Check sheet for the modelled part. Datum: model origin and axes. Units: mm. Round coordinates to 2 decimals unless told otherwise and drop trailing zeros. Loops run counter-clockwise (first coordinate to the right, second up) from the corner with the lowest first, then second, coordinate; pieces in that order, holes last. Notation, with made-up numbers: (74, -40) -> (116, -40) arc R11 ccw to (116, -36) -> close; hole circle Ø4 at (6, 60.25). An arc over 180 degrees is marked (long way). One line per item, written item: value. Start each with the question number.
1. Cross-section at A-A on y = -41.05. Record the cut outline in (x, z), then the cut area to 3 significant figures.
2. Go/stop test with a flat-tipped pin: pin 1 (2.5 mm diameter, centred on x = 5, y = -41.05, fed in from -Z). Record where the tip stops, or that it passes through.
3. Cross-section at C-C on x = 50. Record the cut outline in (y, z), then the cut area to 3 significant figures.
4. Material ranges on L1, parallel to Y at x = 32.55, z = 0.85; L2, parallel to X at y = -76.1, z = 1.15; L3, parallel to Y at x = 21, z = 0.6, recorded low to high.
5. Cross-section at B-B on x = 60.1. Record the cut outline in (y, z).
6. Cross-section at D-D on x = 29. Record the cut outline in (y, z).
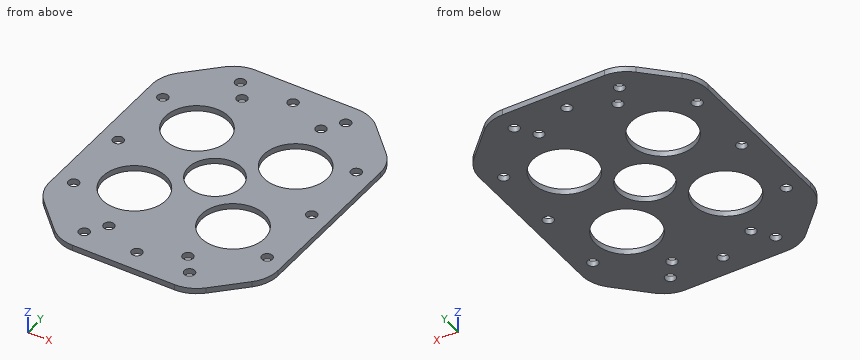
from build123d import *

# Parameters (mm, degrees)
IZIM1_R                     = 9
IZIM1_R_2                   = 7.55
IZIM1_R_3                   = 1.5
Y_KSEKLIK_EKSTR_ZYON1_DEPTH = 1.6


with BuildPart() as part:
    # Çizim1 → Yükseklik-Ekstrüzyon1 (new body)
    with BuildSketch(Plane.XY):
        with BuildLine():
            Line((2.928932188, -10.971067812), (10.971067812, -2.928932188))
            ThreePointArc((10.971067812, -2.928932188), (14.2153013, -0.761204675), (18.042135624, 0))
            Line((18.042135624, 0), (47.057864376, 0))
            ThreePointArc((47.057864376, 0), (50.8846987, -0.761204675), (54.128932188, -2.928932188))
            Line((54.128932188, -2.928932188), (62.171067812, -10.971067812))
            ThreePointArc((62.171067812, -10.971067812), (64.338795325, -14.2153013), (65.1, -18.042135624))
            Line((65.1, -18.042135624), (65.1, -64.057864376))
            ThreePointArc((65.1, -64.057864376), (64.338795325, -67.8846987), (62.171067812, -71.128932188))
            Line((62.171067812, -71.128932188), (54.128932188, -79.171067812))
            ThreePointArc((54.128932188, -79.171067812), (50.8846987, -81.338795325), (47.057864376, -82.1))
            Line((47.057864376, -82.1), (18.042135624, -82.1))
            ThreePointArc((18.042135624, -82.1), (14.2153013, -81.338795325), (10.971067812, -79.171067812))
            Line((10.971067812, -79.171067812), (2.928932188, -71.128932188))
            ThreePointArc((2.928932188, -71.128932188), (0.761204675, -67.8846987), (0, -64.057864376))
            Line((0, -64.057864376), (0, -18.042135624))
            ThreePointArc((0, -18.042135624), (0.761204675, -14.2153013), (2.928932188, -10.971067812))
        make_face()
        with Locations((18.5, -27)):
            Circle(IZIM1_R, mode=Mode.SUBTRACT)
        with Locations((46.6, -27)):
            Circle(IZIM1_R, mode=Mode.SUBTRACT)
        with Locations((18.5, -55.1)):
            Circle(IZIM1_R, mode=Mode.SUBTRACT)
        with Locations((46.6, -55.1)):
            Circle(IZIM1_R, mode=Mode.SUBTRACT)
        with Locations((32.55, -41.05)):
            Circle(IZIM1_R_2, mode=Mode.SUBTRACT)
        with Locations((32.55, -6)):
            Circle(IZIM1_R_3, mode=Mode.SUBTRACT)
        with Locations((47.55, -6)):
            Circle(IZIM1_R_3, mode=Mode.SUBTRACT)
        with Locations((43.8, -11.2)):
            Circle(IZIM1_R_3, mode=Mode.SUBTRACT)
        with Locations((17.55, -6)):
            Circle(IZIM1_R_3, mode=Mode.SUBTRACT)
        with Locations((21.3, -11.2)):
            Circle(IZIM1_R_3, mode=Mode.SUBTRACT)
        with Locations((5, -21.05)):
            Circle(IZIM1_R_3, mode=Mode.SUBTRACT)
        with Locations((60.1, -21.05)):
            Circle(IZIM1_R_3, mode=Mode.SUBTRACT)
        with Locations((5, -41.05)):
            Circle(IZIM1_R_3, mode=Mode.SUBTRACT)
        with Locations((60.1, -41.05)):
            Circle(IZIM1_R_3, mode=Mode.SUBTRACT)
        with Locations(Location((60.1, -61.05, 0), (0, 0, 180))):
            Circle(IZIM1_R_3, mode=Mode.SUBTRACT)
        with Locations(Location((32.55, -76.1, 0), (0, 0, 180))):
            Circle(IZIM1_R_3, mode=Mode.SUBTRACT)
        with Locations(Location((47.55, -76.1, 0), (0, 0, 180))):
            Circle(IZIM1_R_3, mode=Mode.SUBTRACT)
        with Locations(Location((43.8, -70.9, 0), (0, 0, 180))):
            Circle(IZIM1_R_3, mode=Mode.SUBTRACT)
        with Locations(Location((21.3, -70.9, 0), (0, 0, 180))):
            Circle(IZIM1_R_3, mode=Mode.SUBTRACT)
        with Locations(Location((17.55, -76.1, 0), (0, 0, 180))):
            Circle(IZIM1_R_3, mode=Mode.SUBTRACT)
        with Locations(Location((5, -61.05, 0), (0, 0, 180))):
            Circle(IZIM1_R_3, mode=Mode.SUBTRACT)
    extrude(amount=Y_KSEKLIK_EKSTR_ZYON1_DEPTH)


solid = part.part
Taken from the geometry:
1. outline: (0, 0) -> (3.5, 0) -> (3.5, 1.6) -> (0, 1.6) -> close; (6.5, 0) -> (25, 0) -> (25, 1.6) -> (6.5, 1.6) -> close; (40.1, 0) -> (58.6, 0) -> (58.6, 1.6) -> (40.1, 1.6) -> close; (61.6, 0) -> (65.1, 0) -> (65.1, 1.6) -> (61.6, 1.6) -> close
1. area: 70.4 mm2
2. pin 1: passes through
3. outline: (-81.66, 0) -> (-63.43, 0) -> (-63.43, 1.6) -> (-81.66, 1.6) -> close; (-46.77, 0) -> (-35.33, 0) -> (-35.33, 1.6) -> (-46.77, 1.6) -> close; (-18.67, 0) -> (-0.44, 0) -> (-0.44, 1.6) -> (-18.67, 1.6) -> close
3. area: 76.6 mm2
4. L1: y = -82.1 to -77.6, -74.6 to -48.6, -33.5 to -7.5, -4.5 to 0
4. L2: x = 7.9 to 16.05, 19.05 to 31.05, 34.05 to 46.05, 49.05 to 57.2
4. L3: y = -82.1 to -72.37, -69.43 to -63.75, -46.45 to -35.65, -18.35 to -12.67, -9.73 to 0
5. outline: (-73.2, 0) -> (-62.55, 0) -> (-62.55, 1.6) -> (-73.2, 1.6) -> close; (-59.55, 0) -> (-42.55, 0) -> (-42.55, 1.6) -> (-59.55, 1.6) -> close; (-39.55, 0) -> (-22.55, 0) -> (-22.55, 1.6) -> (-39.55, 1.6) -> close; (-19.55, 0) -> (-8.9, 0) -> (-8.9, 1.6) -> (-19.55, 1.6) -> close
6. outline: (-82.1, 0) -> (-47.71, 0) -> (-47.71, 1.6) -> (-82.1, 1.6) -> close; (-34.39, 0) -> (0, 0) -> (0, 1.6) -> (-34.39, 1.6) -> close
